Source: CAD feature listing. Evaluate the final solid. Frame: model axes, mm. A direction names the side the tool comes from. Coordinates: 2 decimals unless noted, no trailing zeros. Write each loop counter-clockwise with the first axis right and the second up, starting at its lowest first coordinate (ties: lowest second). Pieces come first, ordered by that corner, then holes. Notation, with made-up numbers: M 43.25,-12 L 83.25,-12 A23 cw 83.25,8 Z; hole C 89.5,8 d4. An arc over 180 degrees is marked long. Answer as CSV lines item,"result". Start each with the question number.
1. Mould query, pull axis X, two halves, no side actions, for faces 4 (the face through (9, -8, 0)), 5 (the face through (13.56, 4.86, -3.52)), 6 (the face through (2.153, 2.658, 1.231)). Classes: pulls with the +X half, pulls with the -X half, needs draft (parallel to the pull), parting line crosses it, or undercut.
2. Reachability of faces 1 (the face through (13.563, 6.718, -0.925)), 2 (the face through (3.451, 5.775, 0.929)), 3 (the face through (13.563, -6.718, 0.925)) from +Z, -Z, +X, -X, +Y, -Y: full face, straight path, thin tool, end or side. Return the list, or none.
3. Contact query for flat-ended pins moving along their axis: pin 1 Ø6 at (x, z) = (3, 1) entering from +Y; pin 2 Ø4 at (x, y) = (3.5, 6.5) entering from -Z; pin 3 Ø1 at (x, z) = (8.5, -3.5) entering from -Y; pin 4 Ø5 at (x, z) = (11.5, -4.5) entering from +Y. Output: stop coordinate, or through.
4. Line query: probe 1 along Z at (x, y) = (11.75, 4.5); probe 2 along X at (y, z) = (0, -2.8); probe 3 along X at (y, z) = (-2.25, 6.5). Output: solid intervals per line, ascending. Write a range as [from, to].
5. Section A-A on x = 4. Return the cut outline in (y, z).
6. Section B-B on x = 8.25. Return the cut outline in (y, z), plus the area to 3 significant figures.
```python
from build123d import *

# Parameters (mm, degrees)
ESQUISSE1_R                  = 9
ESQUISSE1_R_2                = 2.65
BOSS_EXTRU_1_DEPTH           = 18
ENL_V_MAT_EXTRU_2_DEPTH      = 9
R_P_TITION_CIRCULAIRE1_COUNT = 10
ESQUISSE6_W                  = 3
ESQUISSE6_H                  = 6
ENL_V_MAT_EXTRU_3_DEPTH      = 7
ESQUISSE7_R                  = 2
ENL_V_MAT_EXTRU_4_DEPTH      = 9
R_P_TITION_CIRCULAIRE2_COUNT = 2
R_P_TITION_CIRCULAIRE2_ANGLE = 130


with BuildPart() as part:
    # Esquisse1 → Boss.-Extru.1 (new body)
    with BuildSketch(Plane(origin=(0, 0, 0), x_dir=(0, 0, -1), z_dir=(1, 0, 0))):
        Circle(ESQUISSE1_R)
        Circle(ESQUISSE1_R_2, mode=Mode.SUBTRACT)
    extrude(amount=BOSS_EXTRU_1_DEPTH)

    # Esquisse5 → Enlèv. mat.-Extru.2 (cut)
    with BuildSketch(Plane(origin=(18, 0, 0), x_dir=(0, 0, -1), z_dir=(1, 0, 0))):
        with BuildLine():
            Line((-0.75, 6), (0.75, 6))
            Line((0.75, 6), (1.105, 7.457386359))
            Line((1.105, 7.457386359), (2.579613997, 8.622388974))
            ThreePointArc((2.579613997, 8.622388974), (0, 9), (-2.579613997, 8.622388974))
            Line((-2.579613997, 8.622388974), (-1.105, 7.457386359))
            Line((-1.105, 7.457386359), (-0.75, 6))
        make_face()
    enl_v_mat_extru_2 = extrude(amount=-ENL_V_MAT_EXTRU_2_DEPTH, mode=Mode.SUBTRACT)

    # Répétition circulaire1: Enlèv. mat.-Extru.2 ×10 about axis
    r_p_tition_circulaire1_axis = Axis((0, 0, 0), (1, 0, 0))
    for i in range(1, R_P_TITION_CIRCULAIRE1_COUNT):
        add(enl_v_mat_extru_2.rotate(r_p_tition_circulaire1_axis, i * 360 / R_P_TITION_CIRCULAIRE1_COUNT), mode=Mode.SUBTRACT)

    # Esquisse6 → Enlèv. mat.-Extru.3 (cut)
    with BuildSketch(Plane.ZY):
        with Locations((-5, 0)):
            Rectangle(ESQUISSE6_W, ESQUISSE6_H)
    enl_v_mat_extru_3 = extrude(amount=-ENL_V_MAT_EXTRU_3_DEPTH, mode=Mode.SUBTRACT)

    # Esquisse7 → Enlèv. mat.-Extru.4 (cut)
    with BuildSketch(Plane(origin=(0, 0, -9), x_dir=(-1, 0, 0), z_dir=(0, 0, -1))):
        with Locations((-4, 0)):
            Circle(ESQUISSE7_R)
    enl_v_mat_extru_4 = extrude(amount=-ENL_V_MAT_EXTRU_4_DEPTH, mode=Mode.SUBTRACT)

    # Répétition circulaire2: Enlèv. mat.-Extru.3, Enlèv. mat.-Extru.4 ×2 about axis
    r_p_tition_circulaire2_axis = Axis((0, 0, 0), (1, 0, 0))
    for i in range(1, R_P_TITION_CIRCULAIRE2_COUNT):
        add(enl_v_mat_extru_3.rotate(r_p_tition_circulaire2_axis, i * R_P_TITION_CIRCULAIRE2_ANGLE / (R_P_TITION_CIRCULAIRE2_COUNT - 1)), mode=Mode.SUBTRACT)
        add(enl_v_mat_extru_4.rotate(r_p_tition_circulaire2_axis, i * R_P_TITION_CIRCULAIRE2_ANGLE / (R_P_TITION_CIRCULAIRE2_COUNT - 1)), mode=Mode.SUBTRACT)


solid = part.part
```
Values:
1,face 4,"pulls with the +X half"
1,face 5,"needs draft"
1,face 6,"undercut"
2,face 1,"+X, +Y"
2,face 2,"-X"
2,face 3,"+X, -Y"
3,pin 1,"y = 9"
3,pin 2,"z = -7.79"
3,pin 3,"y = -8.49"
3,pin 4,"y = 8.62"
4,probe 1,"[-7.17, -4.24], [-4.01, 4.01], [4.24, 7.17]"
4,probe 2,"[0, 2], [6, 18]"
4,probe 3,"[0, 9]"
5,outline,"M -3,-6.5 L -3,-3.5 L -2,-3.5 L -2,-1.74 A2.65 cw 0.05,2.65 L 1.4,3.78 L 0.75,4.55 L 3.05,6.48 L 3.69,5.71 L 5.44,7.17 A9 ccw long -2,-8.77 L -2,-6.5 Z; M 2,-8.77 A9 ccw 8.01,4.11 L 6.26,2.65 L 6.91,1.88 L 4.61,-0.05 L 3.97,0.72 L 2.62,-0.41 A2.65 cw 2,-1.74 L 2,-3.5 L 3,-3.5 L 3,-6.5 L 2,-6.5 Z"
6,outline,"C 0,0 d18; hole C 0,0 d5.3"
6,area,"232 mm²"
